Autodesk Inventor part; units mm, degrees
ref_plane "YZ Plane" through (0, 0, 0) normal (1, 0, 0) x (0, 1, 0)
ref_plane "XZ Plane" through (0, 0, 0) normal (0, 1, 0) x (-1, 0, 0)
ref_plane "XY Plane" through (0, 0, 0) normal (0, 0, 1) x (1, 0, 0)
sketch "Sketch1" plane through (0, 0, 0) normal (0, 0, 1) x (1, 0, 0)
  line L0 (-46.6309, 64.3185) -> (53.3691, 64.3185)
  line L1 (53.3691, 64.3185) -> (53.3691, -35.6815)
  line L2 (53.3691, -35.6815) -> (-46.6309, -35.6815)
  line L3 (-46.6309, -35.6815) -> (-46.6309, 64.3185)
  point P0 (0, 0)
  dimension "d0" = 100
  dimension "d1" = 100
extrude "Extrusion1" add sketch "Sketch1" along normal blind 20
sketch "Sketch2" plane through (0, 0, 20) normal (0, 0, 1) x (1, 0, 0)
  line L0 (-14.1309, 31.8185) -> (20.8691, 31.8185)
  line L1 (20.8691, 31.8185) -> (20.8691, 15.5685)
  line L2 (20.8691, 15.5685) -> (-14.1309, 15.5685)
  line L3 (-14.1309, 15.5685) -> (-14.1309, 31.8185)
  line L4 (-14.1309, 15.5685) -> (20.8691, 15.5685)
  line L5 (20.8691, 15.5685) -> (20.8691, 13.0685)
  line L6 (20.8691, 13.0685) -> (-14.1309, 13.0685)
  line L7 (-14.1309, 13.0685) -> (-14.1309, 15.5685)
  line L8 (-14.1309, 13.0685) -> (20.8691, 13.0685)
  line L9 (20.8691, 13.0685) -> (20.8691, -3.1815)
  line L10 (20.8691, -3.1815) -> (-14.1309, -3.1815)
  line L11 (-14.1309, -3.1815) -> (-14.1309, 13.0685)
  line L12 (53.3691, 64.3185) -> (-46.6309, 64.3185)
  line L13 (-46.6309, -35.6815) -> (53.3691, -35.6815)
  line L14 (53.3691, -35.6815) -> (53.3691, 64.3185)
  line L15 (-46.6309, 64.3185) -> (-46.6309, -35.6815)
  point P0 (0, 0)
  dimension "d4" = 2.5
  dimension "d5" = 16.25
  dimension "d6" = 16.25
  dimension "d7" = 32.5
  dimension "d8" = 32.5
  dimension "d9" = 32.5
  dimension "d10" = 32.5
  dimension "d11" = 48.75
extrude "Extrusion2" add sketch "Sketch2" along normal blind 140 contours L0 L1 L2 L3
sketch "Sketch3" plane through (-14.1309, 15.5685, 20) normal (0, -1, 0) x (1, 0, 0)
  circle A0 centre (17.5, 120) radius 7.5
  line L0 (-32.5, 0) -> (67.5, 0)
  line L1 (35, 0) -> (35, 140)
  point P0 (14.1309, -20)
  dimension "d14" = 120
  dimension "d15" = 15
  dimension "d16" = 17.5
extrude "Extrusion3" cut sketch "Sketch3" against normal blind 150
sketch "Sketch4" plane through (0, 0, 20) normal (0, 0, 1) x (1, 0, 0)
  point P0 (0, 0)
sketch "Sketch5" plane through (0, 0, 20) normal (0, 0, 1) x (1, 0, 0)
  line L0 (-14.1309, 15.6081) -> (20.8691, 15.6081)
  line L1 (20.8691, 15.6081) -> (20.8691, 13.1081)
  line L2 (20.8691, 13.1081) -> (-14.1309, 13.1081)
  line L3 (-14.1309, 13.1081) -> (-14.1309, 15.6081)
  line L4 (-14.1309, 31.8185) -> (-14.1309, 15.5685)
  point P0 (0, 0)
  dimension "d19" = 35
  dimension "d20" = 2.5
  dimension "d21" = 0
extrude "Extrusion4" add sketch "Sketch5" along normal blind 120
sketch "Sketch6" plane through (-14.1309, 13.1081, 20) normal (0, -1, 0) x (1, 0, 0)
  circle A0 centre (17.9369, 120) radius 12.75
  line L0 (-32.5, 0) -> (67.5, 0)
  point P0 (14.1309, -20)
  dimension "d24" = 120
  dimension "d25" = 25.5
extrude "Extrusion5" cut sketch "Sketch6" against normal blind 2.5
sketch "Sketch7" plane through (0, 0, 20) normal (0, 0, 1) x (1, 0, 0)
  line L0 (-14.1309, 15.5685) -> (-14.1309, 13.1081)
  line L1 (-14.1309, 13.1081) -> (20.8691, 13.1081)
  line L2 (20.8691, 13.1081) -> (20.8691, -3.1419)
  line L3 (20.8691, -3.1419) -> (-14.1309, -3.1419)
  line L4 (-14.1309, -3.1419) -> (-14.1309, 13.1081)
  point P0 (0, 0)
  dimension "d28" = 16.25
  dimension "d29" = 35
extrude "Extrusion6" add sketch "Sketch7" along normal blind 140
sketch "Sketch8" plane through (-14.1309, -3.1419, 20) normal (0, -1, 0) x (1, 0, 0)
  circle A0 centre (17.5, 120) radius 7.5
  line L0 (35, 0) -> (35, 140)
  line L1 (-32.5, 0) -> (67.5, 0)
  point P0 (14.1309, -20)
  dimension "d33" = 17.5
  dimension "d34" = 15
  dimension "d35" = 120
extrude "Extrusion7" cut sketch "Sketch8" against normal blind 16.25
equation "\"d1\" = d0"
equation "\"d6\" = d5"
equation "\"d8\" = d7"
equation "\"d10\" = d9"
properties part number "linear polariser"
Geometry check sheet. Reference: the model listing, model coordinates, mm. A direction names the side the tool comes from. Coordinates: 2 decimals unless noted, no trailing zeros. Loops run counter-clockwise (first coordinate to the right, second up) from the corner with the lowest first, then second, coordinate; pieces in that order, holes last. Notation, with made-up numbers: (73.25, 18) - (111.25, 18) arc R27 cw to (111.25, 49) - close; hole circle Ø5 at (15.5, 68.25). An arc over 180 degrees is marked (long way). Use one line per item in the form item = value. Start each with the question number.
Item 1: Mould release check, pull along Y, two halves, no side actions. Record for faces 4 (the face through (3, 31.818, 89)), 5 (the face through (3, 5, 160)), 6 (the face through (4, 15.568, 154)): +Y half, -Y half, draft (parallel to the pull), parting line (faces both ways), or undercut.
Item 2: Section check C-C, the plane z = 64.5. Enter the section's corners in (x, y).
Item 3: Section check D-D, the plane x = 34.5. Enter the section's corners in (y, z).
Item 4: Tool access check on faces 1 (the face through (20.869, 15, 89)), 2 (the face through (4, -3.142, 89)), 3 (the face through (7, 13.108, 147)). Record the directions out of +Z, -Z, +X, -X, +Y, -Y that give a thin tool (end or side, any length) a straight path to the whole face; none if there is none.
Item 5: Thickness scan on probe 1 along Z at (x, y) = (3.5, -2); probe 2 along Y at (x, z) = (-10, 134); probe 3 along Z at (x, y) = (-21, 10). Record the ranges inside material, lowest first.
Item 6: Gauge pin test, flat ends, axial feed: pin 1 (22 mm diameter, centred on x = 3, z = 151, fed in from -Y); pin 2 (17 mm diameter, centred on x = 3.37, z = 140, fed in from +Y); pin 3 (2 mm diameter, centred on x = -2.5, z = 137.5, fed in from -Y); pin 4 (10.5 mm diameter, centred on y = 14.5, z = 82, fed in from +X). Record the tip position at first contact, or that the pin passes through.
Item 7: Section check B-B, the plane z = 129. Enter the section's corners in (x, y).
Item 8: Section check A-A, the plane y = 17.5. Enter the section's corners in (x, z), and give its area (3 significant figures).
Computed:
q1.face_4 = +Y half
q1.face_5 = draft
q1.face_6 = undercut
q2.outline = (-14.13, -3.14) - (20.87, -3.14) - (20.87, 31.82) - (-14.13, 31.82) - close
q3.outline = (-35.68, 0) - (64.32, 0) - (64.32, 20) - (-35.68, 20) - close
q4.face_1 = +Z, +X, +Y, -Y
q4.face_2 = +Z, +X, -X, -Y
q4.face_3 = +Z
q5.probe_1 = 0 to 132.5, 147.5 to 160
q5.probe_2 = -3.14 to 31.82
q5.probe_3 = 0 to 20
q6.pin_1 = -3.14
q6.pin_2 = 31.82
q6.pin_3 = through
q6.pin_4 = 20.87
q7.outline = (-14.13, -3.14) - (20.87, -3.14) - (20.87, 31.82) - (-14.13, 31.82) - close; hole (-2.64, 13.11) - (10.25, 13.11) - (10.25, 15.61) - (-2.64, 15.61) - close
q8.outline = (-46.63, 0) - (53.37, 0) - (53.37, 20) - (20.87, 20) - (20.87, 160) - (-14.13, 160) - (-14.13, 20) - (-46.63, 20) - close; hole circle Ø15 at (3.37, 140)
q8.area = 6,720 mm2
